CAD build for the part. Positions are in the model's coordinates, mm. A direction names the side the tool comes from. Coordinates: 2 decimals unless noted, no trailing zeros. Write each loop counter-clockwise with the first axis right and the second up, starting at its lowest first coordinate (ties: lowest second). Pieces come first, ordered by that corner, then holes. Notation, with made-up numbers: (72.25, 71.25) - (110.25, 71.25) arc R18 cw to (110.25, 105.25) - close; hole circle Ø3 at (45.25, -11.75). An arc over 180 degrees is marked (long way). One line per question, with ' | ' between items. Start each with the question number.
1. Band-saw the part on D-D, the plane y = 34.75. Write the cut outline in (x, z).
2. Band-saw the part on A-A, the plane x = 30.5. Write the cut outline in (y, z).
3. Two-plate mould, pull along Y, no slides. Class faces 1 (the cylindrical face through (60.248, 0.713, 19.72)), 2 (the cylindrical face through (-0.693, 30.243, -1.972)), 3 (the cylindrical face through (31.716, 35.865, -1.972)): +Y half, -Y half, draft (parallel to the pull), parting line (faces both ways), or undercut.
4. Probe line 1 (Y direction, x = 30.5, z = -1.9); line 2 (X direction, y = 10, z = 24.5); line 3 (Z direction, x = 22, y = 12). List the from-to ranges inside material, lowest first.
5. Which spindle directions (+Z, -Z, +X, -X, +Y, -Y) get a long thin tool onto all of the face, cutting with end or side? Do faces 4 (the flat face through (0, 15, 20)), 5 (the cylindrical face through (60, 29, 20)), 6 (the flat face through (31, 29.5, 20)), 7 (the flat face through (30, 0, 20)), 8 (the cylindrical face through (1, 29, 20)). Say none if no direction does.
6. Flat gauge pins, fed straight in: P1, Ø2.5, axis at x = 15, z = 43.5, coming from the -Y side; P2, Ø20, axis at x = 22.5, z = 21.5, coming from the -Y side; P3, Ø1.5, axis at y = 8, z = 44, coming from the -X side. Where does each tip first touch, or does it go through?
7. Band-saw the part on C-C, the plane y = 25. Write the cut outline in (x, z), then the cut area to 3 significant figures.
8. Band-saw the part on B-B, the plane z = 28. Write the cut outline in (x, y), then the cut area to 3 significant figures.
from build123d import *

# Parameters (mm, degrees)
BOSS_EXTRUDE1_DEPTH = 40
SKETCH2_R           = 1.65
BOSS_EXTRUDE2_DEPTH = 4
SKETCH3_W           = 1.094631416
SKETCH3_H           = 5.669527591
SKETCH3_W_2         = 8.149744195
SKETCH3_H_2         = 1.362465731
SKETCH3_W_3         = 8.685881664
SKETCH3_H_3         = 1.155421961
BOSS_EXTRUDE3_DEPTH = 13


with BuildPart() as part:
    # Sketch1 → Boss-Extrude1 (new body)
    with BuildSketch(Plane.XY):
        with BuildLine():
            Line((2.5, 0), (58.5, 0))
            ThreePointArc((58.5, 0), (60.267766953, 0.732233047), (61, 2.5))
            Line((61, 2.5), (61, 27))
            ThreePointArc((61, 27), (60.267766953, 28.767766953), (58.5, 29.5))
            Line((58.5, 29.5), (2.5, 29.5))
            ThreePointArc((2.5, 29.5), (0.732233047, 28.767766953), (0, 27))
            Line((0, 27), (0, 2.5))
            ThreePointArc((0, 2.5), (0.732233047, 0.732233047), (2.5, 0))
        make_face()
    extrude(amount=BOSS_EXTRUDE1_DEPTH)

    # Sketch2 → Boss-Extrude2 (add)
    with BuildSketch(Plane(origin=(0, 0, 0), x_dir=(-1, 0, 0), z_dir=(0, 0, -1))):
        with BuildLine():
            Line((-29.192164894, 39.379309675), (-1.942164894, 31.994508834))
            ThreePointArc((-1.942164894, 31.994508834), (0.721094026, 30.206741606), (1.75, 27.168582256))
            Line((1.75, 27.168582256), (1.75, 2.168582256))
            ThreePointArc((1.75, 2.168582256), (0.71380719, -0.879077922), (-1.965293024, -2.663552674))
            Line((-1.965293024, -2.663552674), (-29.215293024, -9.908438343))
            ThreePointArc((-29.215293024, -9.908438343), (-30.5, -10.076303412), (-31.784706976, -9.908438343))
            Line((-31.784706976, -9.908438343), (-59.034706976, -2.663552674))
            ThreePointArc((-59.034706976, -2.663552674), (-61.71380719, -0.879077922), (-62.75, 2.168582256))
            Line((-62.75, 2.168582256), (-62.75, 27.168582256))
            ThreePointArc((-62.75, 27.168582256), (-61.721094026, 30.206741606), (-59.057835106, 31.994508834))
            Line((-59.057835106, 31.994508834), (-31.807835106, 39.379309675))
            ThreePointArc((-31.807835106, 39.379309675), (-30.5, 39.553383097), (-29.192164894, 39.379309675))
        make_face()
        with Locations((-30.5, 34.75)):
            Circle(SKETCH2_R, mode=Mode.SUBTRACT)
        with Locations((-30.5, -5.076303412)):
            Circle(SKETCH2_R, mode=Mode.SUBTRACT)
    extrude(amount=BOSS_EXTRUDE2_DEPTH)

    # Sketch3 → Boss-Extrude3 (add)
    with BuildSketch(Plane.XY.offset(40)):
        with Locations((8.461320631, 14.1528159)):
            Rectangle(SKETCH3_W, SKETCH3_H)
        with Locations((14.54463445, 8.060284138)):
            Rectangle(SKETCH3_W_2, SKETCH3_H_2)
        with Locations((14.812703184, 21.223135875)):
            Rectangle(SKETCH3_W_3, SKETCH3_H_3)
    extrude(amount=BOSS_EXTRUDE3_DEPTH)


solid = part.part
Filled in:
1) outline: (12.11, -4) - (28.85, -4) - (28.85, 0) - (12.11, 0) - close; (32.15, -4) - (48.89, -4) - (48.89, 0) - (32.15, 0) - close
2) outline: (-10.08, -4) - (-6.73, -4) - (-6.73, 0) - (-10.08, 0) - close; (-3.43, -4) - (33.1, -4) - (33.1, 0) - (29.5, 0) - (29.5, 40) - (0, 40) - (0, 0) - (-3.43, 0) - close; (36.4, -4) - (39.55, -4) - (39.55, 0) - (36.4, 0) - close
3) face 1: -Y half | face 2: +Y half | face 3: undercut
4) line 1: y = -10.08 to -6.73, -3.43 to 33.1, 36.4 to 39.55 | line 2: x = 0 to 61 | line 3: z = -4 to 40
5) face 4: +Z, -X, +Y, -Y | face 5: +Z, +X, +Y | face 6: +Z, +X, -X, +Y | face 7: +Z, +X, -X, -Y | face 8: +Z, -X, +Y
6) P1: stops at y = 7.38 | P2: stops at y = 0 | P3: stops at x = 10.47
7) outline: (-1.75, -4) - (62.75, -4) - (62.75, 0) - (61, 0) - (61, 40) - (0, 40) - (0, 0) - (-1.75, 0) - close | area: 2,700 mm²
8) outline: (0, 2.5) arc R2.5 ccw to (2.5, 0) - (58.5, 0) arc R2.5 ccw to (61, 2.5) - (61, 27) arc R2.5 ccw to (58.5, 29.5) - (2.5, 29.5) arc R2.5 ccw to (0, 27) - close | area: 1,790 mm²
